Autodesk Inventor part; units mm, degrees
ref_plane "YZ Plane" through (0, 0, 0) normal (1, 0, 0) x (0, 1, 0)
ref_plane "XZ Plane" through (0, 0, 0) normal (0, 1, 0) x (-1, 0, 0)
ref_plane "XY Plane" through (0, 0, 0) normal (0, 0, 1) x (1, 0, 0)
sketch "Sketch1" plane through (0, 0, 0) normal (0, 0, 1) x (1, 0, 0)
  circle A0 centre (0, 0) radius 17.5
  dimension "d0" = 35
extrude "Extrusion1" add sketch "Sketch1" along normal mid plane 30
sketch "Sketch2" plane through (0, 0, 0) normal (0, 0, 1) x (1, 0, 0)
  line L0 (0, 0) -> (0, -17.5) construction
  line L1 (0, -17.5) -> (-17.5, -17.5)
  line L2 (-17.5, -17.5) -> (-17.5, -14.5) construction
  line L3 (-17.5, -14.5) -> (-13.5, -14.5)
  line L4 (-13.5, -14.5) -> (-11.1906, -10.5)
  line L5 (0, -17.5) -> (17.5, -17.5)
  line L6 (17.5, -17.5) -> (17.5, -14.5) construction
  line L7 (17.5, -14.5) -> (13.5, -14.5)
  line L8 (13.5, -14.5) -> (11.1906, -10.5)
  line L9 (-11.1906, -10.5) -> (11.1906, -10.5)
  circle A0 centre (0, 0) radius 17.5 construction
  line L10 (0, 0) -> (0, -17.5) construction
  line L11 (0, -17.5) -> (25.1989, -17.5) construction
  line L12 (0, 0) -> (-17.5, 0) construction
  line L13 (-17.5, -14.5) -> (-19.5, -14.5)
  line L14 (-19.5, -14.5) -> (-19.5, -17.5)
  line L15 (-19.5, -17.5) -> (-17.5, -17.5)
  line L16 (17.5, -14.5) -> (19.5, -14.5)
  line L17 (19.5, -14.5) -> (19.5, -17.5)
  line L18 (19.5, -17.5) -> (17.5, -17.5)
  dimension "d4" = 3
  dimension "d5" = 4
  dimension "d6" = 60
  dimension "d16" = 0
  dimension "d17" = 4
  dimension "d18" = 2
  dimension "d31" = 35
  dimension "d32" = 39
extrude "Extrusion2" add sketch "Sketch2" along normal mid plane 20
chamfer "Chamfer1" distance 3 angle 45 2 edges at (-17.5, 0, 15) (-17.5, 0, -15)
sketch "Sketch3" plane through (0, 0, 15) normal (0, 0, 1) x (1, 0, 0)
  circle A0 centre (0, 0) radius 14.5
  circle A1 centre (0, 0) radius 3
  dimension "d12" = 6
extrude "Extrusion3" cut sketch "Sketch3" against normal blind 8 contours A1
sketch "Sketch4" plane through (-19.5, -17.5, 10) normal (0, -1, 0) x (1, 0, 0)
  line L0 (19.5, 0) -> (0, 0) construction
  line L1 (0, 0) -> (0, -20) construction
  line L2 (0, -20) -> (19.5, -20) construction
  line L3 (39, 0) -> (39, -20) construction
  line L4 (2, -22) -> (2, 2) construction
  line L5 (37, -22) -> (37, 2) construction
  line L6 (33, 0) -> (33, -20) construction
  line L7 (7.1902, -20) -> (7.1902, 0) construction
  line L8 (2, -5) -> (37, -5) construction
  line L9 (37, -5) -> (37, -15) construction
  line L10 (37, -15) -> (2, -15) construction
  line L11 (2, -15) -> (2, -5) construction
  line L12 (19.5, -20) -> (39, -20)
  line L13 (39, 0) -> (19.5, 0)
  line L14 (19.5, -20) -> (31.8098, -20) construction
  line L15 (19.5, -20) -> (19.5, 0) construction
  line L16 (22.5, -3) -> (16.5, -3) construction
  line L17 (3.5, -5) -> (35.5, -5) construction
  line L18 (35.5, -5) -> (35.5, -15) construction
  line L19 (35.5, -15) -> (3.5, -15) construction
  line L20 (3.5, -15) -> (3.5, -5) construction
  circle A0 centre (3.5, -5) radius 1.25
  circle A1 centre (3.5, -15) radius 1.25
  circle A2 centre (35.5, -5) radius 1.25
  circle A3 centre (35.5, -15) radius 1.25
  point P0 (19.5, -10)
  dimension "d19" = 5
  dimension "d20" = 5
  dimension "d33" = 16
  dimension "d34" = 16
  dimension "d35" = 2.5
extrude "Extrusion4" cut sketch "Sketch4" against normal up to surface (3 mm away)
fillet "Fillet2" radius 2 4 edges at (-19.5, -16, 10) (19.5, -16, 10) (19.5, -16, -10) (-19.5, -16, -10)
sketch "Sketch5" plane through (-13.5, -14.5, 10) normal (0, 1, 0) x (1, 0, 0)
  arc A0 (-4, 20) -> (-6, 18) centre (-4, 18) ccw
  line L0 (-6, 2) -> (-6, 18)
  arc A1 (-6, 2) -> (-4, 0) centre (-4, 2) ccw
  line L1 (-4, 0) -> (0, 0)
  line L2 (0, 0) -> (0, 20)
  line L3 (0, 20) -> (-4, 20)
  line L4 (31.5, 3.8453) -> (29.5, 2.6906)
  line L5 (29.5, 2.6906) -> (27.5, 3.8453)
  line L6 (27.5, 3.8453) -> (27.5, 6.1547)
  line L7 (27.5, 6.1547) -> (29.5, 7.3094)
  line L8 (29.5, 7.3094) -> (31.5, 6.1547)
  line L9 (31.5, 6.1547) -> (31.5, 3.8453)
  circle A2 centre (-2.5, 5) radius 1.25
  circle A3 centre (-2.5, 15) radius 1.25
  circle A4 centre (29.5, 5) radius 1.25
  circle A5 centre (29.5, 15) radius 1.25
  line L10 (-6, 2) -> (-6, 18)
  line L11 (27.5, 13.8453) -> (27.5, 16.1547)
  line L12 (29.5, 12.6906) -> (27.5, 13.8453)
  line L13 (27.5, 16.1547) -> (29.5, 17.3094)
  line L14 (29.5, 17.3094) -> (31.5, 16.1547)
  line L15 (31.5, 16.1547) -> (31.5, 13.8453)
  line L16 (31.5, 13.8453) -> (29.5, 12.6906)
  line L17 (-4.5, 13.8453) -> (-4.5, 16.1547)
  line L18 (-2.5, 12.6906) -> (-4.5, 13.8453)
  line L19 (-4.5, 16.1547) -> (-2.5, 17.3094)
  line L20 (-2.5, 17.3094) -> (-0.5, 16.1547)
  line L21 (-0.5, 16.1547) -> (-0.5, 13.8453)
  line L22 (-0.5, 13.8453) -> (-2.5, 12.6906)
  line L23 (-4.5, 3.8453) -> (-4.5, 6.1547)
  line L24 (-2.5, 2.6906) -> (-4.5, 3.8453)
  line L25 (-4.5, 6.1547) -> (-2.5, 7.3094)
  line L26 (-2.5, 7.3094) -> (-0.5, 6.1547)
  line L27 (-0.5, 6.1547) -> (-0.5, 3.8453)
  line L28 (-0.5, 3.8453) -> (-2.5, 2.6906)
  point P0 (13.5, 10)
  dimension "d26" = 4
  dimension "d36" = 4
  dimension "d37" = 4
  dimension "d38" = 4
extrude "Extrusion5" add sketch "Sketch5" along normal blind 1.5 contours L4 L5 L6 L7 L8 L9 | A2 | A3 | A4 | A5 | L11 L13 L14 L15 L16 L12 | L17 L19 L20 L21 L22 L18 | L23 L25 L26 L27 L28 L24
sketch "Sketch6" plane through (-17.5, -17.5, -10) normal (0, -1, 0) x (1, 0, 0)
  circle A0 centre (1.5, 15) radius 1.25
  circle A1 centre (33.5, 15) radius 1.25
  circle A2 centre (1.5, 5) radius 1.25
  circle A3 centre (33.5, 5) radius 1.25
  point P0 (17.5, 10)
extrude "Extrusion6" add sketch "Sketch6" along normal mid plane 4
properties part number "Motor1"
Part model, mm, in its own coordinate system. A direction names the side the tool comes from. Round coordinates to 2 decimals unless told otherwise and drop trailing zeros. Loops run counter-clockwise (first coordinate to the right, second up) from the corner with the lowest first, then second, coordinate; pieces in that order, holes last.
Item 1: Mould opens along X. For faces 5 (the face through (-16.99, -13.76, 6.74)), 6 (the face through (0, 0, -15)), 7 (the face through (-16, -15.5, -5)) say: +X half, -X half, draft (parallel to the pull), parting line (faces both ways), or undercut.
Item 2: Drop flat-ended pins along their axis: P1, Ø2, axis at x = -16, z = -5, coming from the +Y side; P2, Ø3, axis at x = 15.5, z = 4.5, coming from the +Y side; P3, Ø6, axis at y = 0.5, z = 1, coming from the -X side. Give the stop position or say it passes through.
Item 3: Cut at B-B, the plane y = 0. Give the cut face in (x, z).
Item 4: Cut at C-C, the plane z = 13.25. Give the cut face in (x, y).
Item 5: Cut at A-A, the plane z = -5. State how many separate pieces and enclosed holes the cut face has, then the cut area to 3 significant figures.
Item 6: 3-axis set-ups, long thin cutter, end or side, ignore diameter. For faces 1 (the face through (16, -13, -5)), 2 (the face through (-16.99, -18.49, 5.76)), 3 (the face through (-16, -14.5, -5)), 4 (the face through (-18, -14, 5)): which of +Z, -Z, +X, -X, +Y, -Y reach the whole face in a straight line?
Item 7: Cut at D-D, the plane z = 1. Give the cut face in (x, y).
Item 8: Drill centre lines: line 1 (Y direction, x = 0, z = 9.75); line 2 (X direction, y = -14, z = -6.5); line 3 (X direction, y = 0.5, z = -11.5). Where is each one in solid material? Low to high.
A:
1. face 5: -X half
1. face 6: draft
1. face 7: undercut
2. P1: stops at y = 9.01
2. P2: stops at y = 10.5
2. P3: stops at x = -17.5
3. outline: (-17.5, -12) - (-14.5, -15) - (14.5, -15) - (17.5, -12) - (17.5, 12) - (14.5, 15) - (3, 15) - (3, 7) - (-3, 7) - (-3, 15) - (-14.5, 15) - (-17.5, 12) - close
4. outline: circle Ø32.5 at (0, 0); hole circle Ø6 at (0, 0)
5. separate pieces: 1
5. enclosed holes: 2
5. area: 1,060 mm2
6. face 1: +Z, -Z, +X
6. face 2: -Y
6. face 3: none
6. face 4: +Z, -Z, -X, +Y
7. outline: (-19.5, -17.5) - (19.5, -17.5) - (19.5, -14.5) - (13.5, -14.5) - (12.31, -12.44) arc R17.5 ccw (long way) to (-12.31, -12.44) - (-13.5, -14.5) - (-19.5, -14.5) - close
8. line 1: y = -17.5 to -3, 3 to 17.5
8. line 2: x = -17.4 to -14.6, -13.21 to 13.21, 14.6 to 17.4
8. line 3: x = -17.49 to 17.49
